from build123d import *

# Parameters (mm, degrees)
F0_W      = 76.2
F0_H      = 76.2
F1_DEPTH  = 76.2
F2_W      = 25.4
F2_H      = 25.4
F3_DEPTH  = 12.7
F4_R      = 12.7
F5_DEPTH  = 12.7
F7_D      = 25.4
F9_DEPTH  = 12.7
F11_DEPTH = 12.7


with BuildPart() as f1:
    # F0 (on Front) → F1 (new body)
    with BuildSketch(Plane.XZ):
        with Locations((-7.868283, -18.790566)):
            Rectangle(F0_W, F0_H)
    extrude(amount=-F1_DEPTH)

    # F2 (on face) → F3 (join)
    with BuildSketch(Plane.XZ):
        with Locations((-7.868283, -18.790566)):
            Rectangle(F2_W, F2_H)
    extrude(amount=F3_DEPTH)

    # F4 (on face) → F5 (join)
    with BuildSketch(Plane.YZ.offset(30.231717)):
        with Locations((38.1, -18.790566)):
            Circle(F4_R)
    extrude(amount=F5_DEPTH)

    # F7 (through all)
    with Locations(Plane.XY.offset(19.309434)):
        with Locations((-7.868283, 38.1)):
            Hole(F7_D / 2)

    # F8 (on face) → F9 (join)
    with BuildSketch(Plane(origin=(-45.968283, 0, 0), x_dir=(0, -1, 0), z_dir=(-1, 0, 0))):
        Polygon((-25.4, -31.490566), (-37.803471, -9.324964), (-54.146989, -28.768456), (-56.435099, -31.490566), align=None)
    extrude(amount=F9_DEPTH)

    # F10 (on face) → F11 (join)
    with BuildSketch(Plane(origin=(0, 76.2, 0), x_dir=(-1, 0, 0), z_dir=(0, 1, 0))):
        Polygon((-4.831717, -9.884035), (-4.831717, -26.389956), (10.866347, -31.490566), (20.568283, -18.136995), (10.866347, -4.783425), align=None)
    extrude(amount=F11_DEPTH)


solid = f1.part
Geometry: final body of the model. Coordinates: model frame, mm. A direction names the side the tool comes from. Give positions to 0.01 mm unless a question says otherwise; leave off trailing zeros. Write each loop counter-clockwise with the first axis right and the second up, starting at its lowest first coordinate (ties: lowest second). Pieces come first, ordered by that corner, then holes.
(1) Cut plane D-D, the plane y = 62. Return loops of the section in (x, z).
(2) First-contact query: P1, Ø14, axis at x = -2.5, y = -9, coming from the +Z side; P2, Ø2, axis at x = 17, z = -24, coming from the +Y side; P3, Ø5, axis at y = 69, z = -18, coming from the -X side. Flat tips, straight axial feed; report the tip coordinate or a pass-through.
(3) Cut plane B-B, the plane x = 3.5. Return loops of the section in (y, z).
(4) Cut plane C-C, the plane y = 32.5. Return loops of the section in (x, z).
(5) Ray query, line 1 (X direction, y = 38, z = 0); line 2 (X direction, y = 38, z = -24); line 3 (Y direction, x = 11, z = 14). Return the intervals inside material, ascending.
(6) Cut plane A-A, the plane z = -47.5. Return loops of the section in (x, y), then the cut area to 3 significant figures.
(7) Access query for faces 4 (the flat face through (4.832, -6, -19)), 5 (the cylindrical face through (36.493, 50.214, -14.976)), 6 (the flat face through (-20.568, -6, -19)), 7 (the flat face through (-15.785, 82.461, -11.554)), 8 (the flat face through (-3.127, 82.461, -7.298)). Directions: +Z, -Z, +X, -X, +Y, -Y. A direction counts if a zero-diameter tool reaches every point of the face in a straight line with its end or side. Return the directions, or none.
(8) Mould query, pull axis X, two halves, no side actions, for faces 1 (the flat face through (-8, 88.9, -18)), 2 (the flat face through (4.832, 82, -18)), 3 (the cylindrical face through (-14.696, 48.809, -19.324)). Classes: released by +X, released by -X, zero draft, split by the parting line, or undercut.
Values follow:
1. outline: (-45.97, -56.89) - (30.23, -56.89) - (30.23, 19.31) - (-45.97, 19.31) - close
2. P1: stops at z = -6.09
2. P2: stops at y = 76.2
2. P3: stops at x = -45.97
3. outline: (-12.7, -31.49) - (0, -31.49) - (0, -56.89) - (32.44, -56.89) - (32.44, 19.31) - (0, 19.31) - (0, -6.09) - (-12.7, -6.09) - close; (43.76, -56.89) - (76.2, -56.89) - (76.2, -26.82) - (88.9, -26.82) - (88.9, -9.45) - (76.2, -9.45) - (76.2, 19.31) - (43.76, 19.31) - close
4. outline: (-58.67, -31.49) - (-45.97, -31.49) - (-45.97, -56.89) - (-19.27, -56.89) - (-19.27, 19.31) - (-45.97, 19.31) - (-45.97, -18.8) - (-58.67, -18.8) - close; (3.53, -56.89) - (30.23, -56.89) - (30.23, -30.19) - (42.93, -30.19) - (42.93, -7.39) - (30.23, -7.39) - (30.23, 19.31) - (3.53, 19.31) - close
5. line 1: x = -45.97 to -20.57, 4.83 to 30.23
5. line 2: x = -58.67 to -20.57, 4.83 to 42.93
5. line 3: y = 0 to 76.2
6. outline: (-45.97, 0) - (30.23, 0) - (30.23, 76.2) - (-45.97, 76.2) - close; hole circle Ø25.4 at (-7.87, 38.1)
6. area: 5,300 mm2
7. face 4: +Z, -Z, +X, -Y
7. face 5: +X
7. face 6: +Z, -Z, -X, -Y
7. face 7: +Z, -X, +Y
7. face 8: +Z, +X, +Y
8. face 1: zero draft
8. face 2: released by +X
8. face 3: undercut
